```python
from build123d import *

# Parameters (mm, degrees)
SKETCH_1_W          = 110.7
SKETCH_1_H          = 38.85
EXTRUDE_1_DEPTH     = 0.5
CUT_EXTRUDE_1_DEPTH = 110.343655509


with BuildPart() as part:
    # Эскиз1 → Бобышка-Вытянуть1 (new body)
    with BuildSketch(Plane(origin=(0.5, 0, 0), x_dir=(0, -1, 0), z_dir=(-1, 0, 0))):
        with Locations((-45.5, 22.825)):
            Rectangle(SKETCH_1_W, SKETCH_1_H)
    extrude(amount=-EXTRUDE_1_DEPTH)

    # Эскиз3 → Вырез-Вытянуть1 (cut, through all)
    with BuildSketch(Plane.ZY.offset(-0.5)):
        Polygon((30.006561442, -2.853434514), (16.303695676, -2.853435113), (16.303695676, 71.907533256), (30.006561442, 71.907533256), align=None)
    extrude(amount=-CUT_EXTRUDE_1_DEPTH, mode=Mode.SUBTRACT)


solid = part.part
```
Model file for the job. Use its own axes, mm. Give positions to 0.01 mm unless a question says otherwise; leave off trailing zeros. Loops run counter-clockwise (first coordinate to the right, second up) from the corner with the lowest first, then second, coordinate; pieces in that order, holes last. Notation, with made-up numbers: (8.5, 49.5) - (58.5, 49.5) arc R19 ccw to (58.5, 70.5) - close; hole circle Ø11 at (86.25, 61). An arc over 180 degrees is marked (long way). One line per item, written item: value. Start each with the question number.
1. Slice it at A-A (x = 0.9). List the corners of the cut face in (y, z).
2. Slice it at B-B (z = 22.5). List the corners of the cut face in (x, y), plus the area to 3 significant figures.
3. Probe L1, parallel to Y at x = 0.8, z = 29; L2, parallel to Z at x = 0.65, y = 19. List the from-to ranges inside material, lowest first. Write a range as from..to.
Solution:
1. outline: (-9.85, 3.4) - (100.85, 3.4) - (100.85, 42.25) - (-9.85, 42.25) - close; hole (-2.85, 16.3) - (71.91, 16.3) - (71.91, 30.01) - (-2.85, 30.01) - close
2. outline: (0.5, -9.85) - (1, -9.85) - (1, -2.85) - (0.5, -2.85) - close; (0.5, 71.91) - (1, 71.91) - (1, 100.85) - (0.5, 100.85) - close
2. area: 18.0 mm^2
3. L1: y = -9.85..-2.85, 71.91..100.85
3. L2: z = 3.4..16.3, 30.01..42.25
